Autodesk Inventor part; units mm, degrees
ref_plane "YZ Plane" through (0, 0, 0) normal (1, 0, 0) x (0, 1, 0)
ref_plane "XZ Plane" through (0, 0, 0) normal (0, 1, 0) x (-1, 0, 0)
ref_plane "XY Plane" through (0, 0, 0) normal (0, 0, 1) x (1, 0, 0)
sketch "スケッチ1" plane through (0, 0, 0) normal (0, 1, 0) x (-1, 0, 0)
  line L0 (0, 0) -> (-30, 0)
  line L1 (-30, 0) -> (-30, -30)
  line L2 (-30, -30) -> (0, -30)
  line L3 (0, -30) -> (0, 0)
  dimension "d0" = 30
  dimension "d1" = 30
extrude "押し出し1" add sketch "スケッチ1" along normal blind 5
sketch "スケッチ2" plane through (0, 5, 0) normal (0, 1, 0) x (1, 0, 0)
  line L0 (30, 0) -> (30, 30)
  line L1 (30, 30) -> (0, 30)
  line L2 (0, 30) -> (30, 0) construction
  line L3 (30, 30) -> (0, 0) construction
  circle A0 centre (15, 15) radius 16 construction
  point P0 (26.3137, 26.3137)
  point P1 (26.3137, 3.6863)
  point P2 (3.6863, 3.6863)
  point P3 (3.6863, 26.3137)
  point P4 (15, 15)
  dimension "d12" = 32
  dimension "d76" = 0
hole "穴2" at (26.3137, 5, -26.3137) at (26.3137, 5, -3.6863) at (3.6863, 5, -3.6863) at (3.6863, 5, -26.3137) direction (0, -1, 0) diameter 3.2 end through all
sketch "スケッチ3" plane through (0, 5, 0) normal (0, 1, 0) x (1, 0, 0)
  circle A0 centre (26.3137, 3.6863) radius 1.6
  circle A1 centre (3.6863, 3.6863) radius 1.6
  circle A2 centre (3.6863, 26.3137) radius 1.6
  circle A3 centre (26.3137, 26.3137) radius 1.6
  point P0 (0, 0)
hole "穴3" at (26.3137, 5, -3.6863) at (3.6863, 5, -3.6863) at (3.6863, 5, -26.3137) at (26.3137, 5, -26.3137) direction (0, -1, 0) diameter 5.8 depth 3 tip angle 118
sketch "スケッチ4" plane through (0, 5, 0) normal (0, 1, 0) x (1, 0, 0)
  line L0 (0, 30) -> (0, 0)
  line L1 (30, 0) -> (30, 30)
  line L2 (0, 7) -> (30, 7)
  line L3 (30, 7) -> (30, 23)
  line L4 (30, 23) -> (0, 23)
  line L5 (0, 23) -> (0, 7)
  line L6 (0, 0) -> (30, 0)
  point P0 (0, 23)
  dimension "d27" = 16
  dimension "d28" = 7
extrude "押し出し2" add sketch "スケッチ4" along normal blind 35 contours L4 L1 L2 L0
fillet "フィレット6" radius 2 4 edges at (30, 2.5, 0) (0, 2.5, 0) (0, 2.5, -30) (30, 2.5, -30)
sketch "スケッチ8" plane through (0, 5, -7) normal (0, 0, 1) x (1, 0, 0)
  line L0 (0, 35) -> (30, 35)
  line L1 (2, 0) -> (28, 0)
  point P0 (0, -5)
  point P1 (15, 6)
  point P2 (15, 35)
  point P3 (3.089, 0)
  point P4 (23.911, 0)
  dimension "d61" = 6
hole "穴6" at (15, 11, -7) direction (0, 0, -1) diameter 7.8 end through all
fillet "フィレット7" [suppressed]
fillet "フィレット8" radius 0.2 2 edges at (15, 5, -23) (15, 5, -7)
fillet "フィレット9" radius 1 22 edges at (15, 40, -23) (15, 40, -7) (30, 5.0586, -23.0586) (30, 5, -25.6) (29.4142, 5, -29.4142) (15, 5, -30) (0.5858, 5, -29.4142) (0, 5, -25.6) (0, 5.0586, -23.0586) (0, 22.6, -23) (30, 22.6, -23) (0, 5.0586, -6.9414) (0, 5, -4.4) (0.5858, 5, -0.5858) (15, 5, 0) (29.4142, 5, -0.5858) (30, 5, -4.4) (30, 5.0586, -6.9414) (30, 22.6, -7) (0, 22.6, -7) (0, 40, -15) (30, 40, -15)
fillet "フィレット10" [suppressed]
sketch "スケッチ10" plane through (29, 5.2, -23) normal (0, 0, -1) x (-1, 0, 0)
  line L0 (0, 34.8) -> (28, 34.8) construction
  circle A0 centre (14, 5.8) radius 3.9 construction
  line L1 (14, 34.8) -> (14, 5.8) construction
  arc A1 (9, 31) -> (0, 22) centre (9, 22) ccw construction
  line L2 (14, 5.8) -> (14, 32.2764) construction
  circle A2 centre (14, 5.8) radius 20 construction
  point P0 (29, -5.2)
  point P1 (9, 32)
  point P2 (19, 32)
  point P3 (14, 25.8)
  point P4 (-1, 32)
  point P5 (29, 32)
  dimension "d85" = 40
  dimension "d84" = 0
hole "穴7" at (15, 31, -23) direction (0, 0, 1) diameter 7.8 end through all
properties part number "NewPart2_for_shoulder"
Build history of the part. All positions in model axes, mm. Coordinates: 2 decimals unless noted, no trailing zeros. Order: outer loops, then holes, each group sorted by start corner. A loop starts at its lowest first (then second) coordinate and runs counter-clockwise, first axis right, second up. Notation, with made-up numbers: M 49.25,-30 L 103.25,-30 A12 cw 103.25,-19 Z; hole C 44,-4 d5. An arc over 180 degrees is marked long. One line per question, with ' | ' between items. Start each with the question number.
Q1. Saw through at A-A (x = 15). List the corners of the cut face in (y, z).
Q2. Two-plate mould, pull along Z, no slides. Class faces 1 (the face through (24.96, 0.6, -2.83)), 2 (the face through (27.707, 4.715, -0.301)), 3 (the face through (0.6, 2.03, -29.43)): +Z half, -Z half, draft (parallel to the pull), parting line (faces both ways), or undercut.
Q3. Saw through at C-C (y = 31). List the corners of the cut face in (x, z).
Q4. Saw through at B-B (z = -20). List the corners of the cut face in (x, y), then the cut area to 3 significant figures.
Q5. Probe L1, parallel to Y at x = 15, z = -16.25; L2, parallel to X at y = 31, z = -10; L3, parallel to Z at x = 19, y = 15. List the from-to ranges inside material, lowest first. Write a range as from..to.
Q6. Flat gauge pins, fed straight in: pin 1 Ø0.8 at (x, z) = (28.5, -1.5) entering from +Y; pin 2 Ø10 at (x, y) = (15, 31) entering from -Z; pin 3 Ø3.5 at (x, z) = (26.31, -3.69) entering from +Y; pin 4 Ø7 at (x, y) = (15, 11) entering from -Z. Where does each tip first touch, or does it go through?
Q7. Saw through at D-D (y = 17.5). List the corners of the cut face in (x, z), then the cut area to 3 significant figures.
Check values:
1) outline: M 0,-30 L 4,-30 A1 ccw 5,-29 L 5,-23.2 A0.2 cw 5.2,-23 L 7.1,-23 L 7.1,-7 L 5.2,-7 A0.2 cw 5,-6.8 L 5,-1 A1 ccw 4,0 L 0,0 Z; M 14.9,-23 L 27.1,-23 L 27.1,-7 L 14.9,-7 Z; M 34.9,-23 L 39,-23 A1 ccw 40,-22 L 40,-8 A1 ccw 39,-7 L 34.9,-7 Z
2) face 1: undercut | face 2: +Z half | face 3: -Z half
3) outline: M 0,-22 A1 ccw 1,-23 L 11.1,-23 L 11.1,-7 L 1,-7 A1 ccw 0,-8 Z; M 18.9,-23 L 29,-23 A1 ccw 30,-22 L 30,-8 A1 ccw 29,-7 L 18.9,-7 Z
4) outline: M 0,0 L 30,0 L 30,39 A1 ccw 29,40 L 1,40 A1 ccw 0,39 Z; hole C 15,11 d7.8; hole C 15,31 d7.8 | area: 1,100 mm2
5) L1: y = 0..7.1, 14.9..27.1, 34.9..40 | L2: x = 0..11.1, 18.9..30 | L3: z = -23..-7
6) pin 1: stops at y = 5 | pin 2: stops at z = -23 | pin 3: stops at y = 1.31 | pin 4: passes through
7) outline: M 0,-22 A1 ccw 1,-23 L 29,-23 A1 ccw 30,-22 L 30,-8 A1 ccw 29,-7 L 1,-7 A1 ccw 0,-8 Z | area: 479 mm2
